Can you work these out from the model? Positions are in its coordinate system, mm. Face numbers are marked on the shaded views. A direction names the side the tool comes from. Give positions to 0.01 mm unless a question says otherwise; leave off trailing zeros. Loops run counter-clockwise (first coordinate to the right, second up) from the corner with the lowest first, then second, coordinate; pieces in that order, holes last.
from build123d import *

# Parameters (mm, degrees)
SKETCH1_R           = 6.5
BASEHEAD_DEPTH      = 8
SKETCH2_R           = 4
BASEBODY_DEPTH      = 80
HEXAGONSOCKET_DEPTH = 4
TOPFILLET_R         = 1
CHAMFER1_SIZE       = 0.4
LPATTERN10_COUNT    = 34
LPATTERN10_PITCH    = 0.8118


with BuildPart() as part:
    # Sketch1 → BaseHead (new body)
    with BuildSketch(Plane(origin=(0, 0, 0), x_dir=(0, 0, -1), z_dir=(1, 0, 0))):
        Circle(SKETCH1_R)
    extrude(amount=BASEHEAD_DEPTH)

    # Sketch2 → BaseBody (add)
    with BuildSketch(Plane(origin=(8, 0, 0), x_dir=(0, 0, -1), z_dir=(1, 0, 0))):
        Circle(SKETCH2_R)
    extrude(amount=BASEBODY_DEPTH)

    # Sketch3 → HexagonSocket (cut)
    with BuildSketch(Plane(origin=(0, 0, 0), x_dir=(0, 0, -1), z_dir=(1, 0, 0))):
        Polygon((3.464101615, 0), (1.732050808, 3), (-1.732050808, 3), (-3.464101615, 0), (-1.732050808, -3), (1.732050808, -3), align=None)
    extrude(amount=HEXAGONSOCKET_DEPTH, mode=Mode.SUBTRACT)

    # Sketch4 → Cut-Revolve1 (revolve, cut)
    with BuildSketch(Plane(origin=(-4.19613823, 0.75, 0), x_dir=(-1, 0, 0), z_dir=(0, 0, 1))):
        Polygon((-8.19613823, 3.75), (-9.928189037, 0.75), (-8.19613823, 0.75), align=None)
    revolve(axis=Axis((0.838992387, 0, 0), (-1, 0, 0)), mode=Mode.SUBTRACT)

    # TopFillet
    topfillet_edges = [part.edges().sort_by_distance(p)[0] for p in [
        (0, 0, 6.5),
    ]]
    fillet(topfillet_edges, radius=TOPFILLET_R)

    # Chamfer1
    chamfer1_edges = [part.edges().sort_by_distance(p)[0] for p in [
        (88, 0, 4),
    ]]
    chamfer(chamfer1_edges, length=CHAMFER1_SIZE)

    # Sketch5 → Cut-Revolve10 (revolve, cut)
    with BuildSketch(Plane.XY):
        Polygon((87.6, 3.414133814), (87.93825, 4), (87.93825, 4.6765), (87.26175, 4.6765), (87.26175, 4), align=None)
    cut_revolve10 = revolve(axis=Axis((0, 0, 0), (1, 0, 0)), mode=Mode.SUBTRACT)

    # LPattern10: Cut-Revolve10 ×34
    with Locations(*[(-i * LPATTERN10_PITCH, 0, 0) for i in range(1, LPATTERN10_COUNT)]):
        add(cut_revolve10, mode=Mode.SUBTRACT)


solid = part.part
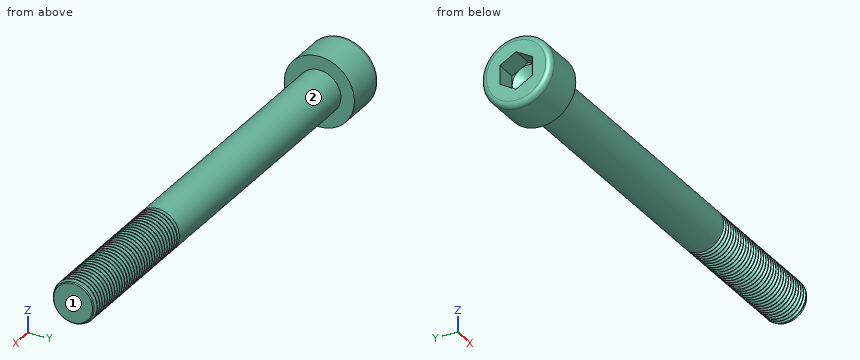
(1) Which directions (+Z, -Z, +X, -X, +Y, -Y) give clear straight access to the entire face, cutting with the end or side of a thin tool? Please do the marked faces 1 and 2.
Returned:
face 1: +Z, -Z, +X, +Y, -Y
face 2: +X
(2) Please list where these lines run through material, in increasing order: probe 1 along X at (y, z) = (-3, 4); probe 2 along Z at (x, y) = (68, 0.25); probe 3 along Y at (x, z) = (33.5, 1.25).
Returned:
probe 1: x = 0 to 8
probe 2: z = -3.61 to 3.61
probe 3: y = -3.8 to 3.8
(3) Suppose I cut it at A-A on x = 26. List the corners of the cut face in (y, z) for me, plus the area to 3 significant figures.
Returned:
outline: circle Ø8 at (0, 0)
area: 50.3 mm2
(4) Will these pins go through, and if not, where does the flat tip stop? P1, Ø1, axis at x = 43.5, y = -1, coming from the +Z side; P2, Ø1.5, axis at y = -0.5, z = 1.5, coming from the -X side; P3, Ø1.5, axis at x = 49.5, z = 1, coming from the -Y side; P4, Ø1, axis at x = 2, z = 0.5, coming from the -Y side.
Returned:
P1: stops at z = 3.97
P2: stops at x = 4.39
P3: stops at y = -3.99
P4: stops at y = -6.5
